The model under review builds one solid part; all positions refer to its coordinate system, in mm. A direction names the side the tool comes from. Give positions to 0.01 mm unless a question says otherwise; leave off trailing zeros. Order: outer loops, then holes, each group sorted by start corner. A loop starts at its lowest first (then second) coordinate and runs counter-clockwise, first axis right, second up.
```python
from build123d import *

# Parameters (mm, degrees)
SKETCH1_R           = 1.6
BOSS_EXTRUDE1_DEPTH = 10
SKETCH1_3_R         = 1.35
BOSS_EXTRUDE2_DEPTH = 3.25
FILLET1_R           = 1


with BuildPart() as part:
    # Sketch1 → Boss-Extrude1 (new body)
    with BuildSketch(Plane(origin=(0, 0, 0), x_dir=(1, 0, 0), z_dir=(0, 1, 0))):
        with BuildLine():
            Line((-16.971, 21), (16.971, 21))
            ThreePointArc((16.971, 21), (19.092078518, 19.092078518), (21, 16.971))
            Line((21, 16.971), (21, -16.971))
            ThreePointArc((21, -16.971), (19.092078518, -19.092078518), (16.971, -21))
            Line((16.971, -21), (-16.971, -21))
            ThreePointArc((-16.971, -21), (-19.092078518, -19.092078518), (-21, -16.971))
            Line((-21, -16.971), (-21, 16.971))
            ThreePointArc((-21, 16.971), (-19.092078518, 19.092078518), (-16.971, 21))
        make_face()
        with Locations(Location((-15.5, 15.5, 0), (0, 0, 270))):
            Circle(SKETCH1_R, mode=Mode.SUBTRACT)
        with Locations(Location((15.5, 15.5, 0), (0, 0, 270))):
            Circle(SKETCH1_R, mode=Mode.SUBTRACT)
        with Locations(Location((15.5, -15.5, 0), (0, 0, 270))):
            Circle(SKETCH1_R, mode=Mode.SUBTRACT)
        with Locations(Location((-15.5, -15.5, 0), (0, 0, 270))):
            Circle(SKETCH1_R, mode=Mode.SUBTRACT)
        with BuildLine():
            Line((-17.1, 12.962284492), (-17.1, -12.962284492))
            ThreePointArc((-17.1, -12.962284492), (-13.378679656, -13.378679656), (-12.962284492, -17.1))
            Line((-12.962284492, -17.1), (12.962284492, -17.1))
            ThreePointArc((12.962284492, -17.1), (13.378679656, -13.378679656), (17.1, -12.962284492))
            Line((17.1, -12.962284492), (17.1, 12.962284492))
            ThreePointArc((17.1, 12.962284492), (13.378679656, 13.378679656), (12.962284492, 17.1))
            Line((12.962284492, 17.1), (-12.962284492, 17.1))
            ThreePointArc((-12.962284492, 17.1), (-13.378679656, 13.378679656), (-17.1, 12.962284492))
        make_face(mode=Mode.SUBTRACT)
    extrude(amount=BOSS_EXTRUDE1_DEPTH)

    # Sketch1_3 → Boss-Extrude2 (add)
    with BuildSketch(Plane(origin=(0, 0, 0), x_dir=(1, 0, 0), z_dir=(0, 1, 0))):
        with BuildLine():
            ThreePointArc((-12.962284492, 17.1), (-13.378679656, 13.378679656), (-17.1, 12.962284492))
            Line((-17.1, 12.962284492), (-17.1, -12.962284492))
            ThreePointArc((-17.1, -12.962284492), (-13.378679656, -13.378679656), (-12.962284492, -17.1))
            Line((-12.962284492, -17.1), (12.962284492, -17.1))
            ThreePointArc((12.962284492, -17.1), (13.378679656, -13.378679656), (17.1, -12.962284492))
            Line((17.1, -12.962284492), (17.1, 12.962284492))
            ThreePointArc((17.1, 12.962284492), (13.378679656, 13.378679656), (12.962284492, 17.1))
            Line((12.962284492, 17.1), (-12.962284492, 17.1))
        make_face()
        with Locations(Location((-8.000195426, -8.000195426, 0), (0, 0, 90))):
            Circle(SKETCH1_3_R, mode=Mode.SUBTRACT)
        with BuildLine():
            ThreePointArc((-9.350195426, 5.546745259), (-6.020296439, 6.019905586), (-5.547136112, 9.349804574))
            Line((-5.547136112, 9.349804574), (5.546745259, 9.349804574))
            ThreePointArc((5.546745259, 9.349804574), (6.019905586, 6.019905586), (9.349804574, 5.546745259))
            Line((9.349804574, 5.546745259), (9.349804574, -5.547136112))
            ThreePointArc((9.349804574, -5.547136112), (6.019905586, -6.020296439), (5.546745259, -9.350195426))
            Line((5.546745259, -9.350195426), (-5.547136112, -9.350195426))
            ThreePointArc((-5.547136112, -9.350195426), (-6.020296439, -6.020296439), (-9.350195426, -5.547136112))
            Line((-9.350195426, -5.547136112), (-9.350195426, 5.546745259))
        make_face(mode=Mode.SUBTRACT)
        with Locations(Location((7.999804574, -8.000195426, 0), (0, 0, 90))):
            Circle(SKETCH1_3_R, mode=Mode.SUBTRACT)
        with Locations(Location((-8.000195426, 7.999804574, 0), (0, 0, 90))):
            Circle(SKETCH1_3_R, mode=Mode.SUBTRACT)
        with Locations(Location((7.999804574, 7.999804574, 0), (0, 0, 90))):
            Circle(SKETCH1_3_R, mode=Mode.SUBTRACT)
    extrude(amount=BOSS_EXTRUDE2_DEPTH)

    # Fillet1
    fillet1_edges = [part.edges().sort_by_distance(p)[0] for p in [
        (12.962284492, 6.625, 17.1),
        (17.1, 6.625, 12.962284492),
        (17.1, 6.625, -12.962284492),
        (12.962284492, 6.625, -17.1),
        (-12.962284492, 6.625, -17.1),
        (-17.1, 6.625, -12.962284492),
        (-17.1, 6.625, 12.962284492),
        (-12.962284492, 6.625, 17.1),
        (5.546745259, 1.625, -9.349804574),
        (9.349804574, 1.625, -5.546745259),
        (9.349804574, 1.625, 5.547136112),
        (5.546745259, 1.625, 9.350195426),
        (-5.547136112, 1.625, 9.350195426),
        (-9.350195426, 1.625, 5.547136112),
        (-9.350195426, 1.625, -5.546745259),
        (-5.547136112, 1.625, -9.349804574),
    ]]
    fillet(fillet1_edges, radius=FILLET1_R)


solid = part.part
```
Item 1: Take a section at C-C (x = 11). Give the boundary of the cut face in (y, z).
Values found:
outline: (0, -21) - (10, -21) - (10, -17.1) - (3.25, -17.1) - (3.25, 17.1) - (10, 17.1) - (10, 21) - (0, 21) - close
Item 2: Take a section at A-A (x = 3). Give the boundary of the cut face in (y, z).
Values found:
outline: (0, -21) - (10, -21) - (10, -17.1) - (3.25, -17.1) - (3.25, -9.35) - (0, -9.35) - close; (0, 9.35) - (3.25, 9.35) - (3.25, 17.1) - (10, 17.1) - (10, 21) - (0, 21) - close
Item 3: Take a section at D-D (y = 1.75). Give the number of separate pieces and of enclosed holes in the cut face, and give its area (3 significant figures).
Values found:
separate pieces: 1
enclosed holes: 9
area: 1,390 mm2
Item 4: For line 1 (X direction, y = 5.75, z = -15.5); line 2 (X direction, y = 8.25, z = -9), list the stretches that pass through material, from the lowest coordinate up.
Values found:
line 1: x = -21 to -17.1, -13.9 to -12.5, 12.5 to 13.9, 17.1 to 21
line 2: x = -21 to -17.1, 17.1 to 21
Item 5: For faces 1 (the cylindrical face through (12.296, 6.672, -16.761)), 2 (the cylindrical face through (-4.963, 1.648, -9.015)), 3 (the flat face through (-21, 5, 0)), list the 3-axis set-ups (+Z, -Z, +X, -X, +Y, -Y) from which the entire face can be reached by the end or side of a thin tool; tool diameter is ignored.
Values found:
face 1: +Y
face 2: +Y, -Y
face 3: +Z, -Z, -X, +Y, -Y
Item 6: Take a section at B-B (y = 4). Give the boundary of the cut face in (x, z), and give its area (3 significant figures).
Values found:
outline: (-21, -16.97) arc R27 ccw to (-16.97, -21) - (16.97, -21) arc R27 ccw to (21, -16.97) - (21, 16.97) arc R27 ccw to (16.97, 21) - (-16.97, 21) arc R27 ccw to (-21, 16.97) - close; hole circle Ø3.2 at (-15.5, -15.5); hole (-17.1, -11.55) arc R1 ccw to (-15.95, -12.53) arc R3 cw to (-12.53, -15.95) arc R1 ccw to (-11.55, -17.1) - (11.55, -17.1) arc R1 ccw to (12.53, -15.95) arc R3 cw to (15.95, -12.53) arc R1 ccw to (17.1, -11.55) - (17.1, 11.55) arc R1 ccw to (15.95, 12.53) arc R3 cw to (12.53, 15.95) arc R1 ccw to (11.55, 17.1) - (-11.55, 17.1) arc R1 ccw to (-12.53, 15.95) arc R3 cw to (-15.95, 12.53) arc R1 ccw to (-17.1, 11.55) - close; hole circle Ø3.2 at (-15.5, 15.5); hole circle Ø3.2 at (15.5, -15.5); hole circle Ø3.2 at (15.5, 15.5)
area: 610 mm2
Item 7: Draft analysis for pull direction Z (two halves, no side actions). For faces 4 (the flat face through (-10, 0, 0)), 5 (the cylindrical face through (19.12, 4.93, 19.064)), 6 (the cylindrical face through (-6.04, 1.6, -6)), 7 (the cylindrical face through (6, 1.6, -6.04)), state which applies: released by +Z, released by -Z, zero draft, split by the parting line, or undercut.
Values found:
face 4: zero draft
face 5: released by +Z
face 6: undercut
face 7: undercut
Item 8: Clearance check with a flat-ended pin moving along its axis: pin 1 Ø6 at (x, z) = (-4, -6) entering from +Y. State where the tip first meets the part, or that it passes through.
Values found:
pin 1: stops at y = 3.25
